from build123d import *

# Parameters (mm, degrees)
SKETCH1_R           = 3.81
BOSS_EXTRUDE1_DEPTH = 2.54


with BuildPart() as part:
    # Sketch1 → Boss-Extrude1 (new body)
    with BuildSketch(Plane.XY):
        with BuildLine():
            Line((-101.6, 0), (-101.6, -177.8))
            Line((-101.6, -177.8), (-50.8, -177.8))
            Line((-50.8, -177.8), (-50.8, 0))
            ThreePointArc((-50.8, 0), (0, 50.8), (50.8, 0))
            Line((50.8, 0), (50.8, -25.4))
            Line((50.8, -25.4), (101.6, 0))
            ThreePointArc((101.6, 0), (0, 101.6), (-101.6, 0))
        make_face()
        with Locations((0, 76.2)):
            Circle(SKETCH1_R, mode=Mode.SUBTRACT)
        with Locations((74.66369609, 15.224075871)):
            Circle(SKETCH1_R, mode=Mode.SUBTRACT)
        with Locations((49.478172332, 57.951276627)):
            Circle(SKETCH1_R, mode=Mode.SUBTRACT)
        with Locations((-46.234392701, 60.570792727)):
            Circle(SKETCH1_R, mode=Mode.SUBTRACT)
        with Locations((-76.2, 17.081132641)):
            Circle(SKETCH1_R, mode=Mode.SUBTRACT)
        with Locations((-76.2, -22.74822838)):
            Circle(SKETCH1_R, mode=Mode.SUBTRACT)
        with Locations((-76.2, -48.14822838)):
            Circle(SKETCH1_R, mode=Mode.SUBTRACT)
        with Locations((-76.2, -73.54822838)):
            Circle(SKETCH1_R, mode=Mode.SUBTRACT)
        with Locations((-76.2, -98.94822838)):
            Circle(SKETCH1_R, mode=Mode.SUBTRACT)
        with Locations((-76.2, -124.34822838)):
            Circle(SKETCH1_R, mode=Mode.SUBTRACT)
        with Locations((-76.2, -149.74822838)):
            Circle(SKETCH1_R, mode=Mode.SUBTRACT)
    extrude(amount=BOSS_EXTRUDE1_DEPTH)


solid = part.part
Can you work these out from the model? Positions are in its coordinate system, mm. Give positions to 0.01 mm unless a question says otherwise; leave off trailing zeros. Loops run counter-clockwise (first coordinate to the right, second up) from the corner with the lowest first, then second, coordinate; pieces in that order, holes last. Notation, with made-up numbers: (30.5, 81.5) -> (71.5, 81.5) arc R18 ccw to (71.5, 90.5) -> close; hole circle Ø10 at (-10, 83). An arc over 180 degrees is marked (long way). Write item = value, one per line.
1) Suppose I cut it at C-C on z = 2.1. Give the number of separate pieces and of enclosed holes in the cut face, then the cut area to 3 significant figures.
Check result:
separate_pieces = 1
enclosed_holes = 11
area = 21,300 mm2
2) Suppose I cut it at A-A on x = 0. Write out the boundary of the cut face in (y, z).
Check result:
outline = (50.8, 0) -> (72.39, 0) -> (72.39, 2.54) -> (50.8, 2.54) -> close; (80.01, 0) -> (101.6, 0) -> (101.6, 2.54) -> (80.01, 2.54) -> close
3) Will this pin go through, and if not, where does the flat tip stop? pin 1 (0.8 mm diameter, centred on y = -54.5, z = 1, fed in from +X).
Check result:
pin_1 = -50.8
4) Thinking about a two-plate mould opening in X: for faces 1 (the flat face through (-47, 26, 0)), 2 (the cylindrical face through (-77.026, -51.868, 1.252)), 3 (the cylindrical face through (2.234, 101.575, 1.252)), 4 (the cylindrical face through (-79.008, 19.656, 1.252)), which applies, released by +X, released by -X, zero draft, split by the parting line, or undercut?
Check result:
face_1 = zero draft
face_2 = undercut
face_3 = split by the parting line
face_4 = undercut
5) Suppose I cut it at B-B on y = 76.2. Write out the boundary of the cut face in (x, z), then the cut area to 3 significant figures.
Check result:
outline = (-67.2, 0) -> (-3.81, 0) -> (-3.81, 2.54) -> (-67.2, 2.54) -> close; (3.81, 0) -> (67.2, 0) -> (67.2, 2.54) -> (3.81, 2.54) -> close
area = 322 mm2
6) I need wall thicknesses on L1, parallel to X at y = 14, z = 1.65; L2, parallel to X at y = -149.5, z = 1.2; L3, parallel to X at y = -64, z = 1.7. Which ranges of each line are inside material? Lowest first, please. Write a range as from..to.
Check result:
L1 = -100.63..-78.44, -73.96..-48.83, 48.83..71.06, 78.27..100.63
L2 = -101.6..-80, -72.4..-50.8
L3 = -101.6..-50.8
